Verification items for this drawing (mm, ordinates from the low corner). Coordinates: 2 decimals unless noted, no trailing zeros. Write each loop counter-clockwise with the first axis right and the second up, starting at its lowest first coordinate (ties: lowest second). Pieces come first, ordered by that corner, then holes.
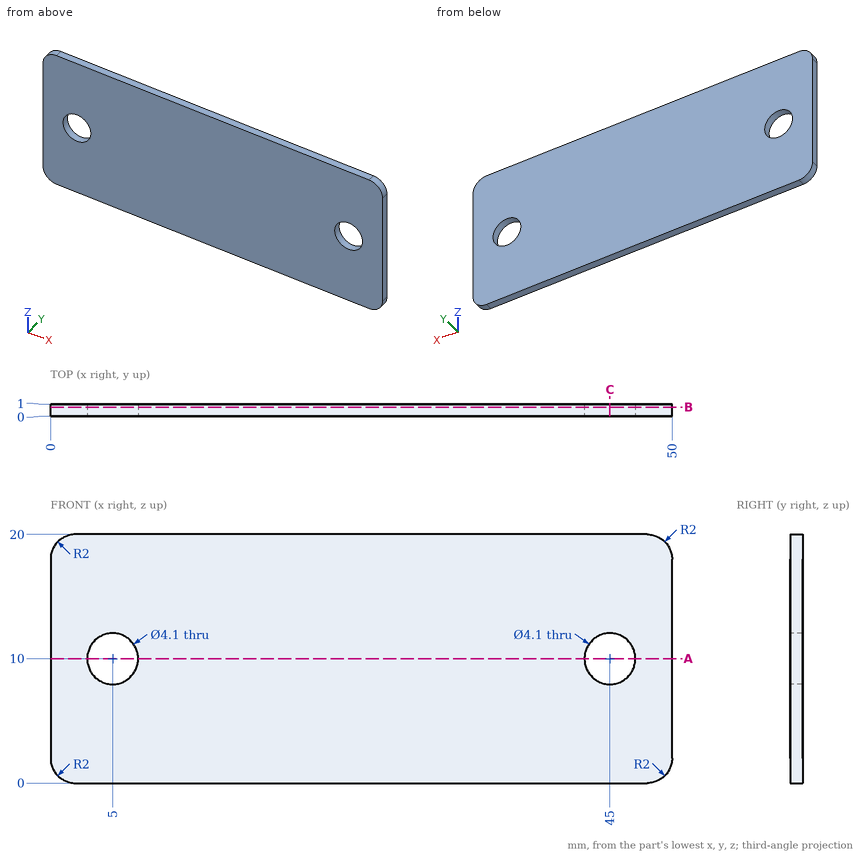
1. Sectioned sample at A-A, the plane z = 10. Record the boundary of the cut face in (x, y), and give its area (3 significant figures).
Computed values:
outline: (0, 0) - (2.95, 0) - (2.95, 1) - (0, 1) - close; (7.05, 0) - (42.95, 0) - (42.95, 1) - (7.05, 1) - close; (47.05, 0) - (50, 0) - (50, 1) - (47.05, 1) - close
area: 41.8 mm2
2. Sectioned sample at C-C, the plane x = 45. Record the boundary of the cut face in (y, z).
Computed values:
outline: (0, 0) - (1, 0) - (1, 7.95) - (0, 7.95) - close; (0, 12.05) - (1, 12.05) - (1, 20) - (0, 20) - close
3. Sectioned sample at B-B, the plane y = 0.75. Record the boundary of the cut face in (x, z), and give its area (3 significant figures).
Computed values:
outline: (0, 2) arc R2 ccw to (2, 0) - (48, 0) arc R2 ccw to (50, 2) - (50, 18) arc R2 ccw to (48, 20) - (2, 20) arc R2 ccw to (0, 18) - close; hole circle Ø4.1 at (5, 10); hole circle Ø4.1 at (45, 10)
area: 970 mm2
4. Thickness scan on line 1 along X through (y, z) = (0.55, 10); line 2 along Z through (x, y) = (5, 0.4); line 3 along X through (y, z) = (0.3, 8.75). Record the ranges inside material, lowest first.
Computed values:
line 1: x = 0 to 2.95, 7.05 to 42.95, 47.05 to 50
line 2: z = 0 to 7.95, 12.05 to 20
line 3: x = 0 to 3.38, 6.62 to 43.38, 46.62 to 50
